from build123d import *

# Parameters (mm, degrees)
F3_D     = 5
F3_DEPTH = 18
F3_TIP   = 1.5021515476
F5_D     = 5
F5_DEPTH = 18
F5_TIP   = 1.5021515476


with BuildPart() as f1:
    # F0 (on Front) → F1 (revolve)
    with BuildSketch(Plane.XZ):
        Polygon((7.5, 80), (2, 80), (2, 65), (0, 65), (0, 15), (2, 15), (2, 0), (7.5, 0), align=None)
    revolve(axis=Axis((0, 0, 48.5607869923), (0, 0, 1)))

    # F3
    with Locations(Plane.XY.offset(80)):
        with Locations((0, 0)):
            Hole(F3_D / 2, depth=F3_DEPTH)
            with Locations((0, 0, -(F3_DEPTH + F3_TIP / 2))):  # 118° drill point
                Cone(0, F3_D / 2, F3_TIP, mode=Mode.SUBTRACT)

    # F5
    with Locations(Plane(origin=(0, 0, 0), x_dir=(1, 0, 0), z_dir=(0, 0, -1))):
        with Locations((0, 0)):
            Hole(F5_D / 2, depth=F5_DEPTH)
            with Locations((0, 0, -(F5_DEPTH + F5_TIP / 2))):  # 118° drill point
                Cone(0, F5_D / 2, F5_TIP, mode=Mode.SUBTRACT)


solid = f1.part
Geometry check sheet. Reference: the model listing, model coordinates, mm. A direction names the side the tool comes from. Round coordinates to 2 decimals unless told otherwise and drop trailing zeros. Write each loop counter-clockwise with the first axis right and the second up, starting at its lowest first coordinate (ties: lowest second). Pieces come first, ordered by that corner, then holes. Notation, with made-up numbers: (59, -37.5) -> (96, -37.5) arc R17 cw to (96, -30.5) -> close; hole circle Ø5 at (-17.5, 1). An arc over 180 degrees is marked (long way). One line per item, written item: value. Start each with the question number.
(1) Go/stop test with flat-tipped pins: pin 1 Ø1 at (x, z) = (2.5, 57.5) entering from +Y; pin 2 Ø8 at (x, z) = (4.5, 47.5) entering from -Y; pin 3 Ø3 at (x, y) = (0, 0) entering from +Z. Record where each tip stops, or that it passes through.
(2) Access from +Z, -Z, +X, -X, +Y, -Y to the whole of each face (thin tool, end or side, straight path). Record for faces 5 (the flat face through (-2, 2, 80)), 6 (the cylindrical face through (0.54, -2.44, 70.87)).
(3) Cross-section at C-C, the plane z = 42. Record the cut outline in (x, y), and give its area (3 significant figures).
(4) Cross-section at A-A, the plane z = 64.5. Record the cut outline in (x, y), and give its area (3 significant figures).
(5) Scan lines: line 1 (Y direction, x = 0, z = 75.25); line 2 (X direction, y = 0.5, z = 26.5); line 3 (Y direction, x = 4.25, z = 37.5). Record each from-to range of solid material in increasing order. Write a range as [from, to].
(6) Draft check along Y on faces 1 (the flat face through (2, 2, 0)), 2 (the cylindrical face through (-7.493, 0.33, 40.56)), 3 (the conical face through (-0.094, 0.424, 19.241)), 4 (the cylindrical face through (0.54, 2.44, 9.13)). Enter one of: +Y half, -Y half, draft (parallel to the pull), parting line (faces both ways), or undercut.
(7) Cross-section at D-D, the plane y = -3.75. Record the cut outline in (x, z), and give its area (3 significant figures).
(8) Cross-section at B-B, the plane x = 6. Record the cut outline in (y, z).
Answer:
1. pin 1: y = 7.23
1. pin 2: y = -7.48
1. pin 3: z = 61.4
2. face 5: +Z, +X, -X, +Y, -Y
2. face 6: +Z
3. outline: circle Ø15 at (0, 0)
3. area: 177 mm²
4. outline: circle Ø15 at (0, 0); hole circle Ø5 at (0, 0)
4. area: 157 mm²
5. line 1: [-7.5, -2.5], [2.5, 7.5]
5. line 2: [-7.48, 7.48]
5. line 3: [-6.18, 6.18]
6. face 1: draft
6. face 2: parting line
6. face 3: undercut
6. face 4: undercut
7. outline: (-6.5, 0) -> (6.5, 0) -> (6.5, 80) -> (-6.5, 80) -> close
7. area: 1,040 mm²
8. outline: (-4.5, 0) -> (4.5, 0) -> (4.5, 80) -> (-4.5, 80) -> close
